```python
from build123d import *

# Parameters (mm, degrees)
SKETCH_R  = 2.5
PAD_DEPTH = 5


with BuildPart() as part:
    # Sketch → Pad (new body)
    with BuildSketch(Plane.XY):
        with BuildLine():
            ThreePointArc((0, 5), (-5, 0), (0, -5))
            Line((0, -5), (119.3, -5))
            ThreePointArc((119.3, -5), (124.3, 0), (119.3, 5))
            Line((0, 5), (119.3, 5))
        make_face()
        Circle(SKETCH_R, mode=Mode.SUBTRACT)
        with BuildLine():
            ThreePointArc((109.3, 2.5), (106.8, 0), (109.3, -2.5))
            Line((109.3, -2.5), (119.3, -2.5))
            ThreePointArc((119.3, -2.5), (121.8, 0), (119.3, 2.5))
            Line((109.3, 2.5), (119.3, 2.5))
        make_face(mode=Mode.SUBTRACT)
    extrude(amount=PAD_DEPTH)


solid = part.part
```
The model under review builds one solid part; all positions refer to its coordinate system, in mm. A direction names the side the tool comes from. Round coordinates to 2 decimals unless told otherwise and drop trailing zeros. Write each loop counter-clockwise with the first axis right and the second up, starting at its lowest first coordinate (ties: lowest second). Pieces come first, ordered by that corner, then holes. Notation, with made-up numbers: (9.5, 12) -> (23.5, 12) arc R8 ccw to (23.5, 16) -> close; hole circle Ø5 at (79, 35.5). An arc over 180 degrees is marked (long way). Use CSV: the item, a comma, the result in double quotes.
Q1. For faces 4 (the cylindrical face through (106.8, 0.1, 2.5)), 5 (the flat face through (59, -5, 2)), list the 3-axis set-ups (+Z, -Z, +X, -X, +Y, -Y) from which the entire face can be reached by the end or side of a thin tool; tool diameter is ignored.
Checks:
face 4,"+Z, -Z"
face 5,"+Z, -Z, +X, -X, -Y"
Q2. For pin 1 Ø1.5 at (x, y) = (96, 0) entering from -Z, flat-tipped, find the tip position at first contact; note if it passes through.
Checks:
pin 1,"z = 0"
Q3. Consider section B-B (x = 115.5). Give the boundary of the cut face in (y, z), then the cut area to 3 significant figures.
Checks:
outline,"(-5, 0) -> (-2.5, 0) -> (-2.5, 5) -> (-5, 5) -> close; (2.5, 0) -> (5, 0) -> (5, 5) -> (2.5, 5) -> close"
area,"25.0 mm²"
Q4. To check wall thickness, follow probe 1 along X at (y, z) = (0.25, 2.6); probe 2 along Y at (x, z) = (114.5, 1.5); probe 3 along X at (y, z) = (-0.5, 2.55). State the ranges of each line that lie inside material, in increasing order. Write a range as [from, to].
Checks:
probe 1,"[-4.99, -2.49], [2.49, 106.81], [121.79, 124.29]"
probe 2,"[-5, -2.5], [2.5, 5]"
probe 3,"[-4.97, -2.45], [2.45, 106.85], [121.75, 124.27]"
Q5. Mouldability with a two-part tool opening along X and no side actions: class faces 1 (the cylindrical face through (-5, 0, 2)), 2 (the cylindrical face through (124.3, -0.1, 2.5)), 3 (the cylindrical face through (-0.54, -2.44, 2.46)) as released by +X, released by -X, zero draft, split by the parting line, or undercut.
Checks:
face 1,"released by -X"
face 2,"released by +X"
face 3,"undercut"
Q6. Consider section C-C (z = 1.25). Give the boundary of the cut face in (x, y).
Checks:
outline,"(0, -5) -> (119.3, -5) arc R5 ccw to (119.3, 5) -> (0, 5) arc R5 ccw to start; hole circle Ø5 at (0, 0); hole (109.3, -2.5) -> (119.3, -2.5) arc R2.5 ccw to (119.3, 2.5) -> (109.3, 2.5) arc R2.5 ccw to start"
Q7. Consider section A-A (y = 0). Give the boundary of the cut face in (x, z).
Checks:
outline,"(-5, 0) -> (-2.5, 0) -> (-2.5, 5) -> (-5, 5) -> close; (2.5, 0) -> (106.8, 0) -> (106.8, 5) -> (2.5, 5) -> close; (121.8, 0) -> (124.3, 0) -> (124.3, 5) -> (121.8, 5) -> close"
